Geometry: final body of the model. Coordinates: model frame, mm. Face numbers are marked on the shaded views. Round coordinates to 2 decimals unless told otherwise and drop trailing zeros. Loops run counter-clockwise (first coordinate to the right, second up) from the corner with the lowest first, then second, coordinate; pieces in that order, holes last. Notation, with made-up numbers: M 21.5,0 L 50.5,0 A35 cw 50.5,35 Z; hole C 70,-36 d10. An arc over 180 degrees is marked long. Answer as a JSON object with one key per item and string values.
```python
from build123d import *

# Parameters (mm, degrees)
F0_W          = 18
F0_H          = 13
F1_DEPTH      = 2.5
F3_DEPTH      = 0.1
F5_R          = 0.5
F6_DEPTH      = 0.5
F8_DEPTH      = 9.001
F8_DEPTH_BACK = 9.001
F10_DEPTH     = 1.6


# Not quite as in the source:
# - a pattern or mirror of a feature is missing from the dataset's text; its kind, count and spacing are read off the source's solid


with BuildPart() as f1:
    # F0 (on Top) → F1 (new body)
    with BuildSketch(Plane.XY):
        Rectangle(F0_W, F0_H)
    extrude(amount=F1_DEPTH)

    # F2 (on face) → F3 (cut)
    with BuildSketch(Plane.XY.offset(2.5)):
        with BuildLine():
            ThreePointArc((7.8, 2.8), (7.067766953, 4.567766953), (5.3, 5.3))
            Line((5.3, 5.3), (-5.3, 5.3))
            ThreePointArc((-5.3, 5.3), (-7.067766953, 4.567766953), (-7.8, 2.8))
            Line((-7.8, 2.8), (-7.8, -2.8))
            ThreePointArc((-7.8, -2.8), (-7.067766953, -4.567766953), (-5.3, -5.3))
            Line((-5.3, -5.3), (5.3, -5.3))
            ThreePointArc((5.3, -5.3), (7.067766953, -4.567766953), (7.8, -2.8))
            Line((7.8, -2.8), (7.8, 2.8))
        make_face()
    extrude(amount=-F3_DEPTH, mode=Mode.SUBTRACT)

    # F5 (on offset) → F6 (join, symmetric)
    with BuildSketch(Plane.YZ.offset(8.1)):
        with Locations((-4.6, -0.15)):
            Circle(F5_R)
    f6 = extrude(amount=F6_DEPTH, both=True)

    # F6_copies: F6 across plane
    add(f6.mirror(Plane(origin=(0, 0, 0), x_dir=(0, 0, -1), z_dir=(-1, 0, 0))))

    # F7 (on Right) → F8 (cut, two sides)
    with BuildSketch(Plane.YZ) as f8_sk:
        with BuildLine():
            Line((-6.5, 0.8), (-6.5, 0))
            Line((-6.5, 0), (-6.175, 0))
            Line((-6.175, 0), (-6.175, 0.5))
            ThreePointArc((-6.175, 0.5), (-6.2628679656, 0.7121320344), (-6.475, 0.8))
            Line((-6.475, 0.8), (-6.5, 0.8))
        make_face()
    f8 = extrude(amount=-F8_DEPTH, mode=Mode.SUBTRACT) + extrude(f8_sk.sketch, amount=F8_DEPTH_BACK, mode=Mode.SUBTRACT)

    # F8_copies: F8 across plane
    add(f8.mirror(Plane.ZX), mode=Mode.SUBTRACT)

    # F9 (on Front) → F10 (join, symmetric)
    with BuildSketch(Plane.XZ):
        Polygon((-9, 1.85), (-9, 2.8), (-9.4, 2.8), (-9.6, 2.6), (-9.6, 1.85), align=None)
    extrude(amount=F10_DEPTH, both=True)


solid = f1.part
```
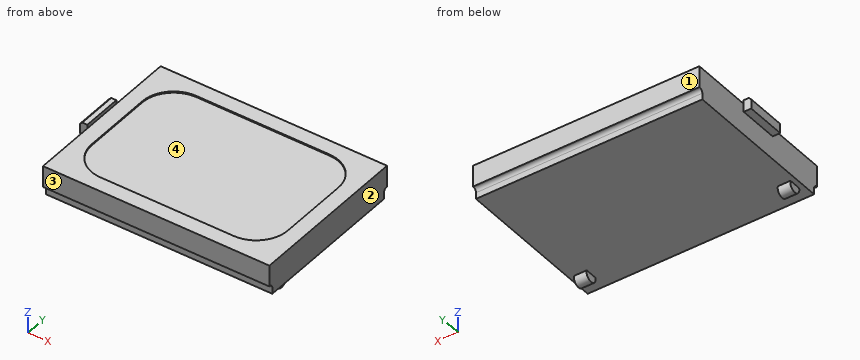
1) Cut plane B-B on y = 1.25. Return the cut outline in (x, z).
Geometry results:
{"outline": "M -9.6,1.85 L -9,1.85 L -9,0 L 9,0 L 9,2.5 L 7.8,2.5 L 7.8,2.4 L -7.8,2.4 L -7.8,2.5 L -9,2.5 L -9,2.8 L -9.4,2.8 L -9.6,2.6 Z"}
2) Cut plane C-C on x = 0.5. Return the cut outline in (y, z) (3 decimals), and give its area (3 significant figures).
Geometry results:
{"outline": "M -6.5,0.8 L -6.475,0.8 A0.3 cw -6.175,0.5 L -6.175,0 L 6.175,0 L 6.175,0.5 A0.3 cw 6.475,0.8 L 6.5,0.8 L 6.5,2.5 L 5.3,2.5 L 5.3,2.4 L -5.3,2.4 L -5.3,2.5 L -6.5,2.5 Z", "area": "31.0 mm2"}
3) Cut plane A-A on z = -0.4. Return the cut outline in (x, y).
Geometry results:
{"outline": "M -8.6,-5.03 L -7.6,-5.03 L -7.6,-4.17 L -8.6,-4.17 Z; M 7.6,-5.03 L 8.6,-5.03 L 8.6,-4.17 L 7.6,-4.17 Z"}
4) Line query: probe 1 along Y at (x, z) = (-1.25, 2.45); probe 2 along Y at (x, z) = (7, 0.1) (3 decimals); probe 3 along Z at (x, y) = (7, -3.5). Output: solid intervals per line, ascending.
Geometry results:
{"probe 1": "-6.5 to -5.3, 5.3 to 6.5", "probe 2": "-6.175 to 6.175", "probe 3": "0 to 2.4"}
5) First-contact query: pin 1 (6.5 mm diameter, centred on x = -2.5, y = 1, fed in from +Z); pin 2 (0.5 mm diameter, centred on x = -9.5, y = 0.5, fed in from -Z); pin 3 (6 mm diameter, centred on x = 1, y = 0.5, fed in from -Z). Flat tips, straight axial feed; report the tip coordinate or a pass-through.
Geometry results:
{"pin 1": "z = 2.4", "pin 2": "z = 1.85", "pin 3": "z = 0"}
6) Pull-direction query (Y, two-part tool) for the marked faces 1, 2, 3 and 4; classes: +Y half, -Y half, draft (parallel to the pull), parting line (faces both ways), or undercut.
Geometry results:
{"face 1": "+Y half", "face 2": "draft", "face 3": "-Y half", "face 4": "undercut"}
7) Cut plane D-D on z = 1.3. Return the cut outline in (x, y), and give its area (3 significant figures).
Geometry results:
{"outline": "M -9,-6.5 L 9,-6.5 L 9,6.5 L -9,6.5 Z", "area": "234 mm2"}
